Could you check a few things on this model? Use its own coordinates, in mm. A direction names the side the tool comes from. Round coordinates to 2 decimals unless told otherwise and drop trailing zeros. Loops run counter-clockwise (first coordinate to the right, second up) from the corner with the lowest first, then second, coordinate; pieces in that order, holes last. Notation, with made-up numbers: (25.5, 64.5) -> (80.5, 64.5) arc R10 cw to (80.5, 70.5) -> close; hole circle Ø10 at (12, 76). An arc over 180 degrees is marked (long way). Write each question's results on one line, items separated by ' | '. Start each with the question number.
1) If I drill on probe 1 along Y at (x, z) = (30, 1.95); probe 2 along Y at (x, z) = (-27, 0.3); probe 3 along Y at (x, z) = (-30.5, 2.25), over which ranges is the centre line in solid material (lowest first)?
2) Imagine slicing it at C-C, the plane y = -73.5. List the corners of the cut face in (x, z) for me, plus the area to 3 significant figures.
3) Imagine slicing it at D-D, the plane x = 15. List the corners of the cut face in (y, z) for me.
4) Which directions (+Z, -Z, +X, -X, +Y, -Y) give clear straight access to the entire face, cutting with the end or side of a thin tool? Please do faces 1 (the flat face through (38, -41.75, 1)), 2 (the flat face through (-5, -83, 1)), 3 (the flat face through (-39, -41.75, 1)), 4 (the flat face through (-23, 8.25, 1)), 5 (the flat face through (40, -11, 1)).
5) Imagine slicing it at A-A, the plane x = 30. List the corners of the cut face in (y, z) for me, plus the area to 3 significant figures.
6) We'd pull the mould along X, two halves only. Please class faces 6 (the flat face through (40, -61, 1)), 7 (the flat face through (1, -36, 3)), 8 (the cylindrical face through (31.908, 0.601, 1.479)): pulls with the +X half, pulls with the -X half, needs draft (parallel to the pull), parting line crosses it, or undercut.
7) For P1, Ø1.5, axis at y = 10, z = 2, coming from the -X side; P2, Ø0.9, axis at x = 38, z = 2, coming from the +Y side; P3, Ø1.5, axis at y = 9.5, z = 2, coming from the +X side; P4, Ø2.5, axis at x = 30, y = 0, coming from the -Z side, each with a flat end and sliding along its axis, tell me the tip position at first contact or that it passes through.
from build123d import *

# Parameters (mm, degrees)
SKETCH1_R           = 2
BOSS_EXTRUDE1_DEPTH = 3


with BuildPart() as part:
    # Sketch1 → Boss-Extrude1 (new body)
    with BuildSketch(Plane.XY):
        Polygon((5, 8.25), (40, 8.25), (40, -31.75), (37, -31.75), (37, -41.75), (40, -41.75), (40, -81.75), (5, -81.75), (5, -84.75), (-5, -84.75), (-5, -81.75), (-40, -81.75), (-40, -41.75), (-37, -41.75), (-37, -31.75), (-40, -31.75), (-40, 8.25), (-5, 8.25), (-5, 11.25), (5, 11.25), align=None)
        with Locations((30, 0)):
            Circle(SKETCH1_R, mode=Mode.SUBTRACT)
        with Locations(Location((30, -73.5, 0), (0, 0, 180))):
            Circle(SKETCH1_R, mode=Mode.SUBTRACT)
        with Locations((-30, -73.5)):
            Circle(SKETCH1_R, mode=Mode.SUBTRACT)
        with Locations(Location((-30, 0, 0), (0, 0, 180))):
            Circle(SKETCH1_R, mode=Mode.SUBTRACT)
    extrude(amount=BOSS_EXTRUDE1_DEPTH)


solid = part.part
Checked values:
1) probe 1: -81.75 to -75.5, -71.5 to -2, 2 to 8.25 | probe 2: -81.75 to 8.25 | probe 3: -81.75 to -75.44, -71.56 to -1.94, 1.94 to 8.25
2) outline: (-40, 0) -> (-32, 0) -> (-32, 3) -> (-40, 3) -> close; (-28, 0) -> (28, 0) -> (28, 3) -> (-28, 3) -> close; (32, 0) -> (40, 0) -> (40, 3) -> (32, 3) -> close | area: 216 mm^2
3) outline: (-81.75, 0) -> (8.25, 0) -> (8.25, 3) -> (-81.75, 3) -> close
4) face 1: +Z, -Z, +X | face 2: +Z, -Z, -X, -Y | face 3: +Z, -Z, -X | face 4: +Z, -Z, -X, +Y | face 5: +Z, -Z, +X, +Y, -Y
5) outline: (-81.75, 0) -> (-75.5, 0) -> (-75.5, 3) -> (-81.75, 3) -> close; (-71.5, 0) -> (-2, 0) -> (-2, 3) -> (-71.5, 3) -> close; (2, 0) -> (8.25, 0) -> (8.25, 3) -> (2, 3) -> close | area: 246 mm^2
6) face 6: pulls with the +X half | face 7: needs draft | face 8: undercut
7) P1: x = -5 | P2: y = 8.25 | P3: x = 5 | P4: through
